Can you work these out from the model? Positions are in its coordinate system, mm. A direction names the side the tool comes from. Give positions to 0.01 mm unless a question says otherwise; leave off trailing zeros. Loops run counter-clockwise (first coordinate to the right, second up) from the corner with the lowest first, then second, coordinate; pieces in that order, holes last. Notation, with made-up numbers: (18.25, 28.25) -> (48.25, 28.25) arc R20 ccw to (48.25, 58.25) -> close; hole circle Ø6 at (-10, 20). An arc over 180 degrees is marked (long way). Use CSV: the item, a comma, the result in double quotes.
from build123d import *

# Parameters (mm, degrees)
BOSS_EXTRUDE1_DEPTH        = 5
BOSS_EXTRUDE2_DEPTH        = 5
SKETCH10_W                 = 7
SKETCH10_H                 = 7
CUT_EXTRUDE2_DEPTH         = 2.6
SKETCH11_R                 = 2.1
CUT_EXTRUDE3_DEPTH         = 37.99114612
F_3_2_3_2_DIAMETER_HOLE1_D = 3.2


with BuildPart() as part:
    # Sketch1 → Boss-Extrude1 (new body)
    with BuildSketch(Plane(origin=(0, 0, 0), x_dir=(1, 0, 0), z_dir=(0, 1, 0))):
        with BuildLine():
            Line((-196.961550602, 34.729635533), (-187.113473072, 32.993153757))
            ThreePointArc((-187.113473072, 32.993153757), (-190, 0), (-187.113473072, -32.993153757))
            Line((-187.113473072, -32.993153757), (-196.961550602, -34.729635533))
            ThreePointArc((-196.961550602, -34.729635533), (-200, 0), (-196.961550602, 34.729635533))
        make_face()
    extrude(amount=BOSS_EXTRUDE1_DEPTH)

    # Sketch9 → Boss-Extrude2 (add)
    with BuildSketch(Plane(origin=(0, 5, 0), x_dir=(1, 0, 0), z_dir=(0, 1, 0))):
        with BuildLine():
            Line((-199.749843554, 10), (-189.73665961, 10))
            ThreePointArc((-189.73665961, 10), (-190, 0), (-189.73665961, -10))
            Line((-189.73665961, -10), (-199.749843554, -10))
            ThreePointArc((-199.749843554, -10), (-200, 0), (-199.749843554, 10))
        make_face()
    extrude(amount=BOSS_EXTRUDE2_DEPTH)

    # Sketch10 → Cut-Extrude2 (cut)
    with BuildSketch(Plane.ZY.offset(195)):
        with Locations((0, 10)):
            Rectangle(SKETCH10_W, SKETCH10_H)
    extrude(amount=CUT_EXTRUDE2_DEPTH, mode=Mode.SUBTRACT)

    # Sketch11 → Cut-Extrude3 (cut, through all)
    with BuildSketch(Plane.ZY.offset(195)):
        with Locations((0, 10)):
            Circle(SKETCH11_R)
    extrude(amount=CUT_EXTRUDE3_DEPTH, mode=Mode.SUBTRACT)

    # Ø3.2 (3.2) Diameter Hole1 (through all)
    with Locations(Plane(origin=(0, 5, 0), x_dir=(1, 0, 0), z_dir=(0, 1, 0))):
        with Locations((-194.257966128, 16.995369836), (-193.331747968, 25.452607483), (-194.257966128, -16.995369836), (-193.331747968, -25.452607483)):
            Hole(F_3_2_3_2_DIAMETER_HOLE1_D / 2)


solid = part.part
(1) If we section it at D-D, the plane y = 2: Write out the boundary of the cut face in (x, z), then the cut area to 3 significant figures.
Answer sheet:
outline,"(-196.96, -34.73) -> (-187.11, -32.99) arc R190 cw to (-187.11, 32.99) -> (-196.96, 34.73) arc R200 ccw to start; hole circle Ø3.2 at (-194.26, -17); hole circle Ø3.2 at (-194.26, 17); hole circle Ø3.2 at (-193.33, -25.45); hole circle Ø3.2 at (-193.33, 25.45)"
area,"649 mm2"
(2) Will these pins go through, and if not, where does the flat tip stop? pin 1 Ø5 at (x, z) = (-193.33, -25.45) entering from +Y; pin 2 Ø1 at (y, z) = (7.5, -1) entering from +X; pin 3 Ø0.8 at (x, z) = (-197, 0.5) entering from +Y.
Answer sheet:
pin 1,"stops at y = 5"
pin 2,"stops at x = -189.99"
pin 3,"stops at y = 6.5"
(3) Which directions (+Z, -Z, +X, -X, +Y, -Y) give clear straight access to the entire face, cutting with the end or side of a thin tool? Please do faces 4 (the face through (-193, 5, -23)), 5 (the face through (-192.99, 2.47, 17.97)), 6 (the face through (-195, 7, 10)), 7 (the face through (-197.6, 7, 0)).
Answer sheet:
face 4,"-Z, +X, -X, +Y"
face 5,"+Y, -Y"
face 6,"+Z, +X, -X, +Y"
face 7,"+Y"
(4) If we section it at C-C, the plane y = 8.75: Write out the boundary of the cut face in (x, z), then the cut area to 3 significant figures.
Answer sheet:
outline,"(-199.99, -1.69) arc R200 ccw to (-199.75, -10) -> (-189.74, -10) arc R190 cw to (-189.74, 10) -> (-199.75, 10) arc R200 ccw to (-199.99, 1.69) -> (-197.6, 1.69) -> (-197.6, 3.5) -> (-195, 3.5) -> (-195, -3.5) -> (-197.6, -3.5) -> (-197.6, -1.69) -> close"
area,"174 mm2"
(5) We'd pull the mould along X, two halves only. Please class faces 1 (the face through (-198.8, 7.9, 0)), 2 (the face through (-191.97, 2.46, 33.85)), 3 (the face through (-194.81, 2.47, -24.84)): released by +X, released by -X, zero draft, split by the parting line, or undercut.
Answer sheet:
face 1,"zero draft"
face 2,"released by +X"
face 3,"undercut"
(6) If I drill on L1, parallel to Z at x = -194, y = 3.75; L2, parallel to Z at x = -198.5, y = 7.5; L3, parallel to Y at x = -196.25, z = -24, over which ranges is the centre line in solid material (lowest first)? Write a range as from..to.
Answer sheet:
L1,"z = -34.21..-26.91, -24..-18.57, -15.42..15.42, 18.57..24, 26.91..34.21"
L2,"z = -10..10"
L3,"y = 0..5"
(7) If we section it at B-B, the plane z = 0: Write out the boundary of the cut face in (x, y), then the cut area to 3 significant figures.
Answer sheet:
outline,"(-200, 0) -> (-190, 0) -> (-190, 10) -> (-195, 10) -> (-195, 6.5) -> (-197.6, 6.5) -> (-197.6, 7.9) -> (-200, 7.9) -> close"
area,"85.9 mm2"
(8) If we section it at A-A, the plane x = -189: Write out the boundary of the cut face in (y, z).
Answer sheet:
outline,"(0, -33.33) -> (5, -33.33) -> (5, -19.47) -> (0, -19.47) -> close; (0, 19.47) -> (5, 19.47) -> (5, 33.33) -> (0, 33.33) -> close"
